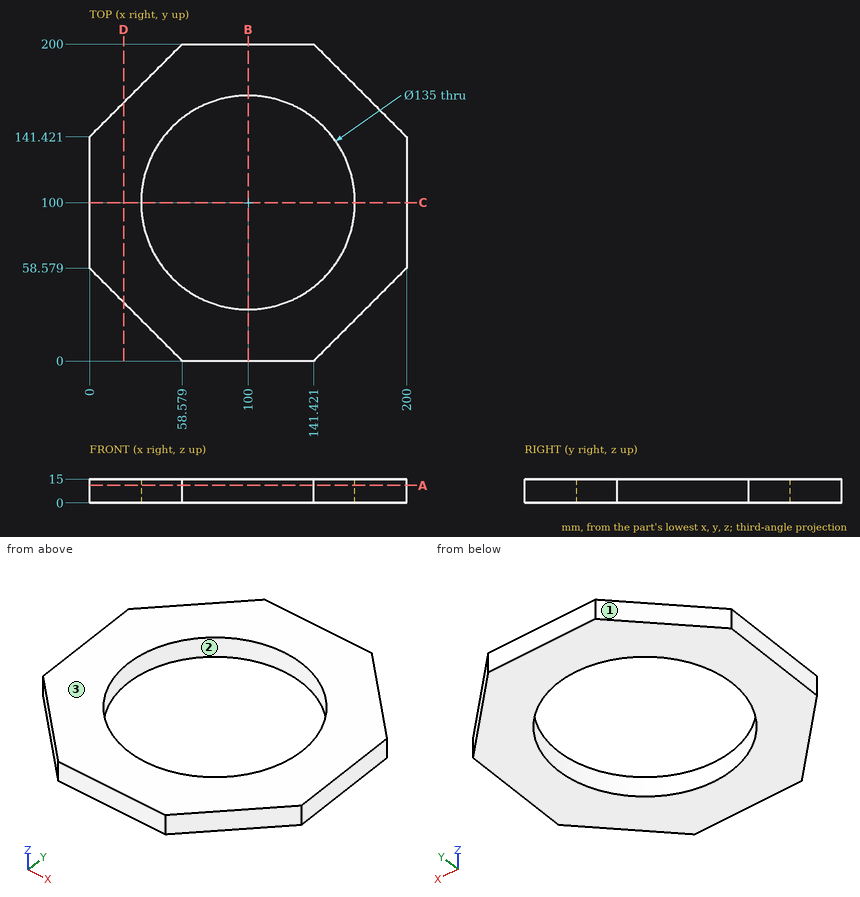
Geometry check sheet. Reference: drawing and pictorial views, mm from the part's lowest x, y, z. Round coordinates to 2 decimals unless told otherwise and drop trailing zeros. Loops run counter-clockwise (first coordinate to the right, second up) from the corner with the lowest first, then second, coordinate; pieces in that order, holes last. Notation, with made-up numbers: (14.25, 69) -> (22.25, 69) arc R23 ccw to (22.25, 81) -> close; hole circle Ø6 at (-37.5, 15.5). An arc over 180 degrees is marked (long way). Answer as a JSON object with one key per item and string values.
Q1. Scan lines: line 1 (Y direction, x = 100, z = 10.5); line 2 (Y direction, x = 136, z = 10.25); line 3 (X direction, y = 49.5, z = 2.5). Record each from-to range of solid material in increasing order. Write a range as from..to.
Data:
{"line 1": "y = 0..32.5, 167.5..200", "line 2": "y = 0..42.9, 157.1..200", "line 3": "x = 9.08..55.21, 144.79..190.92"}
Q2. Draft check along X on the marked faces 1, 2 and 3. Enter one of: pulls with the +X half, pulls with the -X half, needs draft (parallel to the pull), parting line crosses it, or undercut.
Data:
{"face 1": "pulls with the -X half", "face 2": "undercut", "face 3": "needs draft"}
Q3. Section check A-A (z = 11). Record the boundary of the cut face in (x, y), then the cut area to 3 significant figures.
Data:
{"outline": "(0, 58.58) -> (58.58, 0) -> (141.42, 0) -> (200, 58.58) -> (200, 141.42) -> (141.42, 200) -> (58.58, 200) -> (0, 141.42) -> close; hole circle Ø135 at (100, 100)", "area": "18,800 mm2"}
Q4. Go/stop test with flat-tipped pins: P1, Ø1.5, axis at x = 39, z = 13, coming from the +Y side; P2, Ø1, axis at x = 38, z = 4.5, coming from the +Y side; P3, Ø2, axis at y = 163, z = 8.5, coming from the -X side. Record where each tip stops, or that it passes through.
Data:
{"P1": "stops at y = 181.17", "P2": "stops at y = 179.92", "P3": "stops at x = 20.58"}
Q5. Section check B-B (x = 100). Record the boundary of the cut face in (y, z).
Data:
{"outline": "(0, 0) -> (32.5, 0) -> (32.5, 15) -> (0, 15) -> close; (167.5, 0) -> (200, 0) -> (200, 15) -> (167.5, 15) -> close"}
Q6. Section check D-D (x = 21.5). Record the boundary of the cut face in (y, z).
Data:
{"outline": "(37.08, 0) -> (162.92, 0) -> (162.92, 15) -> (37.08, 15) -> close"}
